Build history of the part. All positions in model axes, mm. A direction names the side the tool comes from. Give positions to 0.01 mm unless a question says otherwise; leave off trailing zeros. Order: outer loops, then holes, each group sorted by start corner. A loop starts at its lowest first (then second) coordinate and runs counter-clockwise, first axis right, second up. Notation, with made-up numbers: (-3.75, -29) - (10.25, -29) arc R27 ccw to (10.25, -6) - close; hole circle Ø2 at (85, -7). An arc over 180 degrees is marked (long way). One line per item, written item: value.
```python
from build123d import *

# Parameters (mm, degrees)
SKETCH2_R           = 1.4605
BOSS_EXTRUDE1_DEPTH = 1.5875
FILLET1_R           = 5.08


with BuildPart() as part:
    # Sketch2 → Boss-Extrude1 (new body, symmetric)
    with BuildSketch(Plane(origin=(0, 0, 0), x_dir=(1, 0, 0), z_dir=(0, 1, 0))):
        Polygon((4.445, -34.925), (4.445, -31.75), (6.35, -31.75), (6.35, 31.75), (-6.35, 31.75), (-6.35, -31.75), (-4.445, -31.75), (-4.445, -34.925), align=None)
        with Locations((0, 25.4)):
            Circle(SKETCH2_R, mode=Mode.SUBTRACT)
    extrude(amount=BOSS_EXTRUDE1_DEPTH, both=True)

    # Fillet1
    fillet1_edges = [part.edges().sort_by_distance(p)[0] for p in [
        (6.35, 0, -31.75),
        (-6.35, 0, -31.75),
    ]]
    fillet(fillet1_edges, radius=FILLET1_R)


solid = part.part
```
(1) Slice it at A-A, the plane z = -25.4. Give the cut face in (x, y).
Completed:
outline: (-6.35, -1.59) - (-1.46, -1.59) - (-1.46, 1.59) - (-6.35, 1.59) - close; (1.46, -1.59) - (6.35, -1.59) - (6.35, 1.59) - (1.46, 1.59) - close
(2) Pull direction X, two halves, no side cores. Call faces 1 (the face through (0, 0, 34.925)), 2 (the face through (6.35, 0, 3)), 3 (the face through (0.67, -0.02, -24.1)), 4 (the face through (-6.35, 0, 2)): +X half, -X half, draft (parallel to the pull), parting line (faces both ways), or undercut.
Completed:
face 1: draft
face 2: +X half
face 3: undercut
face 4: -X half
(3) 3-axis set-ups, long thin cutter, end or side, ignore diameter. For faces 5 (the face through (-4.901, 0.022, -30.222)), 6 (the face through (5, 0, 31.75)), 7 (the face through (-4.445, 0, 33)): which of +Z, -Z, +X, -X, +Y, -Y reach the whole face in a straight line?
Completed:
face 5: -Z, -X, +Y, -Y
face 6: +Z, +X, +Y, -Y
face 7: +Z, -X, +Y, -Y
(4) Pin check, flat tips, straight feed: P1, Ø0.6, axis at x = 5.5, y = 0, coming from the +Z side; P2, Ø1.5, axis at x = -2.5, y = 0, coming from the -Z side; P3, Ø1, axis at y = 0, z = 34, coming from the +X side (3 decimals). Stop position of each tip, or through.
Completed:
P1: z = 31.75
P2: z = -31.73
P3: x = 4.445
(5) Drill centre lines: line 1 (X direction, y = 0.5, z = -25.4); line 2 (Z direction, x = -1, y = 0.75) (3 decimals); line 3 (Z direction, x = 0.5, y = 1.4) (3 decimals). Where is each one in solid material? Low to high.
Completed:
line 1: -6.35 to -1.46, 1.46 to 6.35
line 2: -31.75 to -26.464, -24.336 to 34.925
line 3: -31.75 to -26.772, -24.028 to 34.925
(6) Slice it at D-D, the plane x = -5. Give the cut face in (y, z), and give its area (3 significant figures).
Completed:
outline: (-1.59, -30.12) - (1.59, -30.12) - (1.59, 31.75) - (-1.59, 31.75) - close
area: 196 mm²
